from build123d import *

# Parameters (mm, degrees)
SKETCH1_R               = 6
BOSS_EXTRUDE1_DEPTH     = 5
SKETCH2_R               = 3
BOSS_EXTRUDE2_DEPTH     = 2.5
BOSS_EXTRUDE3_DEPTH     = 12
CUT_EXTRUDE1_REACH      = 23.915
CUT_EXTRUDE1_END_RADIUS = 3
SKETCH4_R               = 1.5


with BuildPart() as part:
    # Sketch1 → Boss-Extrude1 (new body)
    with BuildSketch(Plane.XY):
        Circle(SKETCH1_R)
    extrude(amount=BOSS_EXTRUDE1_DEPTH)

    # Sketch2 → Boss-Extrude2 (add)
    with BuildSketch(Plane.XY.offset(5)):
        Circle(SKETCH2_R)
    extrude(amount=BOSS_EXTRUDE2_DEPTH)

    # Sketch3 → Boss-Extrude3 (add)
    with BuildSketch(Plane.XY.offset(7.5)):
        with BuildLine():
            Line((-2.236067977, -2), (2.236067977, -2))
            ThreePointArc((2.236067977, -2), (0, 3), (-2.236067977, -2))
        make_face()
    extrude(amount=BOSS_EXTRUDE3_DEPTH)

    # Cut-Extrude1: up to this cylinder (the profile starts inside it)
    cut_extrude1_end = Plane(origin=(0, 0, 12.5), z_dir=(0, 0, -1)) * Cylinder(CUT_EXTRUDE1_END_RADIUS, 54.83, mode=Mode.PRIVATE)
    # Sketch4 → Cut-Extrude1 (cut, up to the surface)
    with BuildSketch(Plane.XZ.offset(2), mode=Mode.PRIVATE) as cut_extrude1_sk1:
        with Locations(Location((0, 12.5, 0), (0, 0, 270))):
            Circle(SKETCH4_R)
    cut_extrude1_tool1 = extrude(cut_extrude1_sk1.sketch, amount=-CUT_EXTRUDE1_REACH, mode=Mode.PRIVATE) & cut_extrude1_end
    add(cut_extrude1_tool1.solids().sort_by_distance((0, -2, 12.5))[0], mode=Mode.SUBTRACT)


solid = part.part
Build history of the part. All positions in model axes, mm. A direction names the side the tool comes from. Coordinates: 2 decimals unless noted, no trailing zeros. Write each loop counter-clockwise with the first axis right and the second up, starting at its lowest first coordinate (ties: lowest second). Pieces come first, ordered by that corner, then holes.
(1) Cut at B-B on y = 0. List the corners of the cut face in (x, z).
(2) Cut at A-A on x = 0. List the corners of the cut face in (y, z), and give its area (3 significant figures).
(3) Mould opens along Z. For faces 4 (the flat face through (0, 1, 19.5)), 5 (the cylindrical face through (-6, 0, 2)), 6 (the cylindrical face through (-0.575, 0.465, 11.114)) say: pulls with the +Z half, pulls with the -Z half, needs draft (parallel to the pull), parting line crosses it, or undercut.
(4) Cut at D-D on y = -1.5. List the corners of the cut face in (x, z), and give its area (3 significant figures).
(5) Cut at C-C on z = 12.5. List the corners of the cut face in (x, y), and give its area (3 significant figures).
(6) Drill centre lines: line 1 (Z direction, x = 0, y = -1); line 2 (Z direction, x = 3.75, y = -2.75); line 3 (X direction, y = -0.05, z = 12.5). Where is each one in solid material? Low to high.
(7) Pin check, flat tips, straight feed: pin 1 Ø4 at (x, z) = (-3.5, 8.5) entering from -Y; pin 2 Ø6 at (x, z) = (-2.5, 13.5) entering from -Y; pin 3 Ø4 at (y, z) = (4.5, 11.5) entering from +X. Stop position of each tip, or through.
(8) 3-axis set-ups, long thin cutter, end or side, ignore diameter. For faces 1 (the flat face through (0, 0, 0)), 2 (the flat face through (-3, -1, 5)), 3 (the flat face through (0, -2, 15)): which of +Z, -Z, +X, -X, +Y, -Y reach the whole face in a straight line?
Working result:
1. outline: (-6, 0) - (6, 0) - (6, 5) - (3, 5) - (3, 19.5) - (-3, 19.5) - (-3, 5) - (-6, 5) - close; hole circle Ø3 at (0, 12.5)
2. outline: (-6, 0) - (6, 0) - (6, 5) - (3, 5) - (3, 11) - (-2, 11) - (-2, 7.5) - (-3, 7.5) - (-3, 5) - (-6, 5) - close; (-2, 14) - (3, 14) - (3, 19.5) - (-2, 19.5) - close
2. area: 120 mm2
3. face 4: pulls with the +Z half
3. face 5: needs draft
3. face 6: undercut
4. outline: (-5.81, 0) - (5.81, 0) - (5.81, 5) - (2.6, 5) - (2.6, 19.5) - (-2.6, 19.5) - (-2.6, 5) - (-5.81, 5) - close; hole circle Ø3 at (0, 12.5)
4. area: 126 mm2
5. outline: (-2.24, -2) - (-1.5, -2) - (-1.5, 2.6) arc R3 ccw to start; (1.5, -2) - (2.24, -2) arc R3 ccw to (1.5, 2.6) - close
5. area: 10.6 mm2
6. line 1: z = 0 to 11, 14 to 19.5
6. line 2: z = 0 to 5
6. line 3: x = -3 to -1.5, 1.5 to 3
7. pin 1: stops at y = -2.42
7. pin 2: stops at y = -2
7. pin 3: stops at x = 1.66
8. face 1: -Z, +X, -X, +Y, -Y
8. face 2: +Z
8. face 3: +Z, +X, -X, -Y
